Work out the finished part from the listing and answer in its coordinate system (mm). A direction names the side the tool comes from. Give positions to 0.01 mm unless a question says otherwise; leave off trailing zeros. Order: outer loops, then holes, each group sorted by start corner. A loop starts at its lowest first (then second) coordinate and runs counter-clockwise, first axis right, second up. Notation, with made-up numbers: M -32.5,17.5 L 16.5,17.5 A20 ccw 16.5,33.5 Z; hole C -31,55.5 d5. An arc over 180 degrees is marked long. One line per item, written item: value.
Autodesk Inventor part; units mm, degrees
ref_plane "YZ Plane" through (0, 0, 0) normal (1, 0, 0) x (0, 1, 0)
ref_plane "XZ Plane" through (0, 0, 0) normal (0, 1, 0) x (-1, 0, 0)
ref_plane "XY Plane" through (0, 0, 0) normal (0, 0, 1) x (1, 0, 0)
sketch "Sketch1" plane through (0, 0, 0) normal (0, 1, 0) x (-1, 0, 0)
  circle A0 centre (0, 0) radius 14
  dimension "d0" = 28
extrude "Extrusion1" add sketch "Sketch1" along normal blind 2
sketch "Sketch2" plane through (0, 2, 0) normal (0, 1, 0) x (1, 0, 0)
  circle A0 centre (0, 0) radius 12.5
  dimension "d3" = 25
extrude "Extrusion2" add sketch "Sketch2" along normal blind 3.5
sketch "Sketch3" plane through (0, 5.5, 0) normal (0, 1, 0) x (1, 0, 0)
  line L0 (5, -2.8868) -> (0, -5.7735)
  line L1 (0, -5.7735) -> (-5, -2.8868)
  line L2 (-5, -2.8868) -> (-5, 2.8868)
  line L3 (-5, 2.8868) -> (0, 5.7735)
  line L4 (0, 5.7735) -> (5, 2.8868)
  line L5 (5, 2.8868) -> (5, -2.8868)
  point P0 (0, 0)
  point P1 (0, 0)
  dimension "d6" = 10
extrude "Extrusion3" cut sketch "Sketch3" against normal blind 2
sketch "Sketch4" plane through (0, 5.5, 0) normal (0, 1, 0) x (1, 0, 0)
  circle A0 centre (0, 0) radius 1.5
  circle A1 centre (0, 0) radius 7.5 construction
  circle A2 centre (-7.5, 0) radius 1.5
  circle A3 centre (-3.75, -6.4952) radius 1.5
  circle A4 centre (3.75, -6.4952) radius 1.5
  circle A5 centre (7.5, 0) radius 1.5
  circle A6 centre (3.75, 6.4952) radius 1.5
  circle A7 centre (-3.75, 6.4952) radius 1.5
  dimension "d13" = 15
  dimension "d12" = 3
  dimension "d14" = 3
  dimension "d17" = 360
extrude "Extrusion4" cut sketch "Sketch4" against normal through all contours A0 | A2 | A4 | A6
chamfer "Chamfer2" distance 0.25 angle 45 1 edges at (14, 0, 0)
chamfer "Chamfer3" distance 0.25 angle 45 6 edges at (-5, 5.5, 0) (-2.5, 5.5, 4.3301) (2.5, 5.5, 4.3301) (5, 5.5, 0) (2.5, 5.5, -4.3301) (-2.5, 5.5, -4.3301)
properties part number "Shaft2_Joint2" material "ABS Plastic"
(1) Section D-D, the plane y = 4.7 is taken. Give the vertices of the cut face in (x, z), then the cut area to 3 significant figures.
Findings:
outline: C 0,0 d25; hole C -7.5,0 d3; hole M -5,-2.89 L 0,-5.77 L 5,-2.89 L 5,2.89 L 0,5.77 L -5,2.89 Z; hole C 3.75,-6.5 d3; hole C 3.75,6.5 d3
area: 383 mm^2
(2) Section A-A, the plane z = 0 is taken. Give the number of separate pieces and of enclosed holes in the cut face, then the cut area to 3 significant figures.
Findings:
separate pieces: 3
enclosed holes: 0
area: 96.4 mm^2
(3) Determine the mould class of faces 1 (the cylindrical face through (5.136, 2.788, 7.07)), 2 (the flat face through (-2.598, 5.373, 4.416)), 3 (the cylindrical face through (-12.932, 1.113, 5.362)), 4 (the flat face through (0, 0, -3)) for opening direction X: pulls with the +X half, pulls with the -X half, needs draft (parallel to the pull), parting line crosses it, or undercut.
Findings:
face 1: undercut
face 2: undercut
face 3: parting line crosses it
face 4: needs draft
(4) Given P1, Ø0.5, axis at y = 4, z = -1, coming from the -X side; P2, Ø3, axis at x = -10, y = 4, coming from the +Z side; P3, Ø1.5, axis at y = 4, z = -5, coming from the +X side; P4, Ø2.5, axis at x = 0, z = 0, coming from the -Y side, each flat-ended and moving along its own axis, determine where each tip first touches the part or whether it passes through.
Findings:
P1: stops at x = -12.48
P2: stops at z = 9.17
P3: stops at x = 11.76
P4: passes through
(5) Which of the six approach directions +Z, -Z, +X, -X, +Y, -Y give full straight-line access (tool end or side, diameter ignored) to faces 5 (the flat face through (5.4, 5.5, -0.2)), 6 (the flat face through (-2.52, 5.37, -4.46))?
Findings:
face 5: +Z, -Z, +X, -X, +Y
face 6: +Y
(6) Find the intervals of material crossed by probe 1 along X at (y, z) = (2.2, 0); probe 2 along Z at (x, y) = (3.75, 4.1); probe 3 along Y at (x, z) = (11.75, 5), in increasing order. Write a range as from..to.
Findings:
probe 1: x = -12.5..-9, -6..-1.5, 1.5..12.5
probe 2: z = -11.92..-8, -5..-3.61, 3.61..5, 8..11.92
probe 3: y = 0..2
(7) Section B-B, the plane y = 1.2 is taken. Give the vertices of the cut face in (x, z), then the cut area to 3 significant figures.
Findings:
outline: C 0,0 d28; hole C -7.5,0 d3; hole C 0,0 d3; hole C 3.75,-6.5 d3; hole C 3.75,6.5 d3
area: 587 mm^2
